Could you check a few things on this model? Use its own coordinates, in mm. Face numbers are marked on the shaded views. A direction names the side the tool comes from. Give positions to 0.01 mm unless a question says otherwise; leave off trailing zeros. Write each loop counter-clockwise with the first axis right and the second up, starting at its lowest first coordinate (ties: lowest second). Pieces come first, ordered by that corner, then holes. Notation, with made-up numbers: (-15, 34) - (32, 34) arc R19 cw to (32, 66) - close; hole circle Ø11 at (0.5, 66.25). An arc over 180 degrees is marked (long way). Answer in a Markdown table with one row per item.
from build123d import *

# Parameters (mm, degrees)
SKETCH_1_W      = 28
SKETCH_1_H      = 22
SKETCH_1_R      = 1.5
EXTRUDE_1_DEPTH = 3
EXTRUDE_START   = -3
SKETCH_2_W      = 52
SKETCH_2_H      = 15
SKETCH_2_R      = 1.5
EXTRUDE_3_DEPTH = 3
FILLET_1_R      = 3


with BuildPart() as part:
    # 草图1 → 凸台-拉伸1 (new body)
    with BuildSketch(Plane.XY):
        Rectangle(SKETCH_1_W, SKETCH_1_H)
        with Locations((7.5, 5)):
            Circle(SKETCH_1_R, mode=Mode.SUBTRACT)
        with Locations(Location((7.5, -5, 0), (0, 0, 180))):
            Circle(SKETCH_1_R, mode=Mode.SUBTRACT)
        with Locations((-7.5, -5)):
            Circle(SKETCH_1_R, mode=Mode.SUBTRACT)
        with Locations(Location((-7.5, 5, 0), (0, 0, 180))):
            Circle(SKETCH_1_R, mode=Mode.SUBTRACT)
    extrude(amount=EXTRUDE_1_DEPTH)

    # 草图2 → 凸台-拉伸3 (add)
    with BuildSketch(Plane.XY.offset(3).offset(EXTRUDE_START)):
        with Locations((0, -5)):
            Rectangle(SKETCH_2_W, SKETCH_2_H)
        with Locations((20, -5)):
            Circle(SKETCH_2_R, mode=Mode.SUBTRACT)
        with Locations(Location((-20, -5, 0), (0, 0, 180))):
            Circle(SKETCH_2_R, mode=Mode.SUBTRACT)
        with Locations((-7.5, -5)):
            Circle(SKETCH_2_R, mode=Mode.SUBTRACT)
        with Locations(Location((7.5, -5, 0), (0, 0, 180))):
            Circle(SKETCH_2_R, mode=Mode.SUBTRACT)
    extrude(amount=EXTRUDE_3_DEPTH)

    # 圆角1
    fillet_1_edges = [part.edges().sort_by_distance(p)[0] for p in [
        (-14, 2.5, 1.5),
        (-26, 2.5, 1.5),
        (26, 2.5, 1.5),
        (26, -12.5, 1.5),
        (-26, -12.5, 1.5),
        (14, 2.5, 1.5),
        (-14, 11, 1.5),
        (14, 11, 1.5),
    ]]
    fillet(fillet_1_edges, radius=FILLET_1_R)


solid = part.part
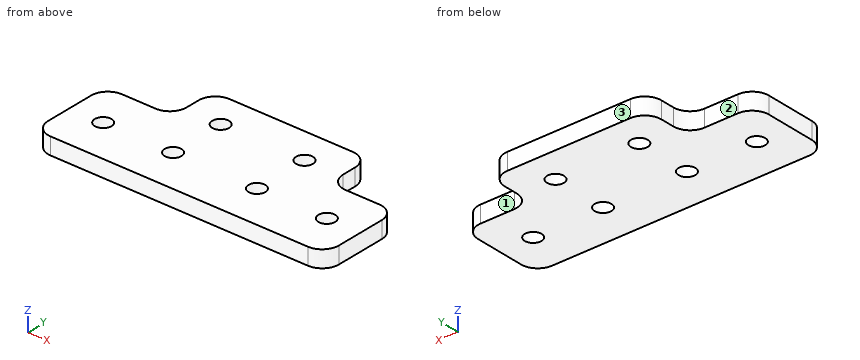
1) Imagine slicing it at C-C (z = 0.7). List the corners of the cut face in (x, y) for me.
Check values:
| item | result |
|---|---|
| outline | (-26, -9.5) arc R3 ccw to (-23, -12.5) - (23, -12.5) arc R3 ccw to (26, -9.5) - (26, -0.5) arc R3 ccw to (23, 2.5) - (17, 2.5) arc R3 cw to (14, 5.5) - (14, 8) arc R3 ccw to (11, 11) - (-11, 11) arc R3 ccw to (-14, 8) - (-14, 5.5) arc R3 cw to (-17, 2.5) - (-23, 2.5) arc R3 ccw to (-26, -0.5) - close; hole circle Ø3 at (-20, -5); hole circle Ø3 at (-7.5, -5); hole circle Ø3 at (-7.5, 5); hole circle Ø3 at (7.5, -5); hole circle Ø3 at (7.5, 5); hole circle Ø3 at (20, -5) |
2) Imagine slicing it at B-B (x = 7.5). List the corners of the cut face in (y, z) for me.
Check values:
| item | result |
|---|---|
| outline | (-12.5, 0) - (-6.5, 0) - (-6.5, 3) - (-12.5, 3) - close; (-3.5, 0) - (3.5, 0) - (3.5, 3) - (-3.5, 3) - close; (6.5, 0) - (11, 0) - (11, 3) - (6.5, 3) - close |
3) If I drill on line 1 (Y direction, x = -7.5, z = 2.8); line 2 (Y direction, x = -20, z = 2.3); line 3 (Y direction, x = -8, z = 0.5), over which ranges is the centre line in solid material (lowest first)?
Check values:
| item | result |
|---|---|
| line 1 | y = -12.5 to -6.5, -3.5 to 3.5, 6.5 to 11 |
| line 2 | y = -12.5 to -6.5, -3.5 to 2.5 |
| line 3 | y = -12.5 to -6.41, -3.59 to 3.59, 6.41 to 11 |
4) Imagine slicing it at D-D (y = 5). List the corners of the cut face in (x, z) for me, then the cut area to 3 significant figures.
Check values:
| item | result |
|---|---|
| outline | (-14.04, 0) - (-9, 0) - (-9, 3) - (-14.04, 3) - close; (-6, 0) - (6, 0) - (6, 3) - (-6, 3) - close; (9, 0) - (14.04, 0) - (14.04, 3) - (9, 3) - close |
| area | 66.3 mm2 |
5) Will these pins go through, and if not, where does the flat tip stop? P1, Ø0.9, axis at x = 21, z = 2, coming from the +Y side; P2, Ø2.5, axis at x = -20, y = -5, coming from the +Z side; P3, Ø1.2, axis at y = 7, z = 2, coming from the +X side.
Check values:
| item | result |
|---|---|
| P1 | stops at y = 2.5 |
| P2 | passes through |
| P3 | stops at x = 14 |
6) Imagine slicing it at A-A (y = -5). List the corners of the cut face in (x, z) for me.
Check values:
| item | result |
|---|---|
| outline | (-26, 0) - (-21.5, 0) - (-21.5, 3) - (-26, 3) - close; (-18.5, 0) - (-9, 0) - (-9, 3) - (-18.5, 3) - close; (-6, 0) - (6, 0) - (6, 3) - (-6, 3) - close; (9, 0) - (18.5, 0) - (18.5, 3) - (9, 3) - close; (21.5, 0) - (26, 0) - (26, 3) - (21.5, 3) - close |
7) On a 3-axis mill with a long thin cutter (end or side, diameter ignored), from which of +Z, -Z, +X, -X, +Y, -Y can I reach the whole of each face in a straight line? I mean the marked faces 1, 2 and 3. Say none if no direction works.
Check values:
| item | result |
|---|---|
| face 1 | +Z, -Z, +X, +Y |
| face 2 | +Z, -Z, -X, +Y |
| face 3 | +Z, -Z, +X, -X, +Y |
